Check sheet for the modelled part. Datum: model origin and axes. Units: mm. A direction names the side the tool comes from. Give positions to 0.01 mm unless a question says otherwise; leave off trailing zeros. Order: outer loops, then holes, each group sorted by start corner. A loop starts at its lowest first (then second) coordinate and runs counter-clockwise, first axis right, second up.
```python
from build123d import *

# Parameters (mm, degrees)
ESQUISSE1_W             = 300
ESQUISSE1_H             = 20
BOSS_EXTRU_1_DEPTH      = 5
ESQUISSE2_R             = 2
ENL_V_MAT_EXTRU_1_DEPTH = 5
ESQUISSE3_W             = 10
ESQUISSE3_H             = 20
BOSS_EXTRU_2_DEPTH      = 35
CONG_1_R                = 10
CONG_2_R                = 10
ESQUISSE4_R             = 1.5
ENL_V_MAT_EXTRU_2_DEPTH = 35
ESQUISSE6_R             = 2.5
ENL_V_MAT_EXTRU_3_DEPTH = 5


# Some blends are built 0.0001 mm under size
with BuildPart() as part:
    # Esquisse1 → Boss.-Extru.1 (new body)
    with BuildSketch(Plane.XY):
        Rectangle(ESQUISSE1_W, ESQUISSE1_H)
    extrude(amount=BOSS_EXTRU_1_DEPTH)

    # Esquisse2 → Enlèv. mat.-Extru.1 (cut)
    with BuildSketch(Plane.XY.offset(5)):
        with Locations((-140, 5)):
            Circle(ESQUISSE2_R)
        with Locations((-140, -5)):
            Circle(ESQUISSE2_R)
        with Locations((-65, 5)):
            Circle(ESQUISSE2_R)
        with Locations((-65, -5)):
            Circle(ESQUISSE2_R)
        with Locations((10, 5)):
            Circle(ESQUISSE2_R)
        with Locations((10, -5)):
            Circle(ESQUISSE2_R)
        with Locations((65, 5)):
            Circle(ESQUISSE2_R)
        with Locations((65, -5)):
            Circle(ESQUISSE2_R)
        with Locations((140, 5)):
            Circle(ESQUISSE2_R)
        with Locations((140, -5)):
            Circle(ESQUISSE2_R)
    extrude(amount=-ENL_V_MAT_EXTRU_1_DEPTH, mode=Mode.SUBTRACT)

    # Esquisse3 → Boss.-Extru.2 (add)
    with BuildSketch(Plane(origin=(0, 0, 0), x_dir=(-1, 0, 0), z_dir=(0, 0, -1))):
        Rectangle(ESQUISSE3_W, ESQUISSE3_H)
    extrude(amount=BOSS_EXTRU_2_DEPTH)

    # Congé1
    # the kernel refuses this fillet: 10 mm, written as the material it adds along each edge
    with BuildSketch(Plane(origin=(5, 10, 0), x_dir=(1, 0, 0), z_dir=(0, -1, 0))) as cong_1_piece_1_section:
        with BuildLine():
            CenterArc((CONG_1_R, -CONG_1_R), CONG_1_R, 90, 90)
            Line((0, -CONG_1_R), (0, 0))
            Line((0, 0), (CONG_1_R, 0))
        make_face()
    cong_1_piece_1 = extrude(amount=20, mode=Mode.PRIVATE)
    cong_1_piece_1 = cong_1_piece_1 - Plane(origin=(10, -5, -2.39791943), x_dir=(1, 0, 0), z_dir=(0, 0, 1)) * Cylinder(2, 80, mode=Mode.PRIVATE)
    cong_1_piece_1 = cong_1_piece_1 - Plane(origin=(10, 5, -2.39791943), x_dir=(1, 0, 0), z_dir=(0, 0, 1)) * Cylinder(2, 80, mode=Mode.PRIVATE)
    add(cong_1_piece_1)
    with BuildSketch(Plane(origin=(-5, -10, 0), x_dir=(-1, 0, 0), z_dir=(0, 1, 0))) as cong_1_piece_2:
        with BuildLine():
            CenterArc((CONG_1_R, -CONG_1_R), CONG_1_R, 90, 90)
            Line((0, -CONG_1_R), (0, 0))
            Line((0, 0), (CONG_1_R, 0))
        make_face()
    extrude(amount=20)

    # Congé2
    cong_2_edges = [part.edges().sort_by_distance(p)[0] for p in [
        (0, -10, -35),
        (0, 10, -35),
    ]]
    fillet(cong_2_edges, radius=CONG_2_R - 0.0001)  # a hair under: the kernel refuses the full size

    # Esquisse4 → Enlèv. mat.-Extru.2 (cut)
    with BuildSketch(Plane.ZY.offset(5)):
        with Locations(Location((-25, 0, 0), (0, 0, 270))):
            Circle(ESQUISSE4_R)
    extrude(amount=-ENL_V_MAT_EXTRU_2_DEPTH, mode=Mode.SUBTRACT)

    # Esquisse6 → Enlèv. mat.-Extru.3 (cut)
    with BuildSketch(Plane(origin=(5, 0, 0), x_dir=(0, 0, -1), z_dir=(1, 0, 0))):
        with Locations(Location((25, 0, 0), (0, 0, 90))):
            Circle(ESQUISSE6_R)
    extrude(amount=-ENL_V_MAT_EXTRU_3_DEPTH, mode=Mode.SUBTRACT)


solid = part.part
```
(1) Release check for a two-part mould opening along Z. For faces 1 (the face through (-150, 0, 2)), 2 (the face through (-2, 0, 5)), 3 (the face through (2.54, -0.33, -22.52)) record: released by +Z, released by -Z, zero draft, split by the parting line, or undercut.
(2) Tool access check on faces 4 (the face through (0, 2, -25)), 5 (the face through (-83, 0, 0)), 6 (the face through (-1, -10, 1)), 7 (the face through (5, 0, -22)). Record the directions out of +Z, -Z, +X, -X, +Y, -Y that give a thin tool (end or side, any length) a straight path to the whole face; none if there is none.
(3) Go/stop test with flat-tipped pins: P1, Ø6.5, axis at x = -140, y = -5, coming from the -Z side; P2, Ø2.5, axis at x = 65, y = 5, coming from the +Z side; P3, Ø6, axis at y = 4, z = -16, coming from the -X side; P4, Ø6, axis at y = 1, z = -25, coming from the +X side. Record where each tip stops, or that it passes through.
(4) Sectioned sample at A-A (z = -16). Enter the section's corners in (x, y), plus the area to 3 significant figures.
(5) Thickness scan on L1, parallel to Y at x = 140, z = 1; L2, parallel to Z at x = -1.3, y = 0; L3, parallel to X at y = 0.5, z = -29.5. Record the ranges inside material, lowest first.
(6) Sectioned sample at B-B (x = -130). Enter the section's corners in (y, z), plus the area to 3 significant figures.
Values follow:
1. face 1: zero draft
1. face 2: released by +Z
1. face 3: undercut
2. face 4: +X
2. face 5: -Z, -X, +Y, -Y
2. face 6: +Z, -Z, +X, -X, -Y
2. face 7: -Z, +X, +Y, -Y
3. P1: stops at z = 0
3. P2: passes through
3. P3: stops at x = -5
3. P4: stops at x = 5
4. outline: (-5, -10) - (5, -10) - (5, 10) - (-5, 10) - close
4. area: 200 mm2
5. L1: y = -10 to -7, -3 to 3, 7 to 10
5. L2: z = -35 to -26.5, -23.5 to 5
5. L3: x = -5 to 5
6. outline: (-10, 0) - (10, 0) - (10, 5) - (-10, 5) - close
6. area: 100 mm2
